from build123d import *

# Parameters (mm, degrees)
MODEL_R         = 9.4
MODEL_R_2       = 2.5
EXTRUDE_1_DEPTH = 6
SKETCH_2_W      = 6.222861065
SKETCH_2_H      = 6.222861065
SKETCH_2_W_2    = 12
SKETCH_2_H_2    = 6
SKETCH_2_W_3    = 11.79
SKETCH_2_H_3    = 6.29
SKETCH_2_W_4    = 6.039723033
SKETCH_2_H_4    = 6.178960273
SKETCH_2_H_5    = 12
SKETCH_2_W_5    = 6
SKETCH_2_H_6    = 6.764977387
EXTRUDE_2_DEPTH = 2


with BuildPart() as part:
    # Model → 凸台-拉伸1 (new body)
    with BuildSketch(Plane.XY):
        Polygon((1072.862228674, 1168.347447046), (1072.862228674, 1127.547447046), (1012.463824187, 1127.108430595), (1012.463824187, 1167.908430595), align=None)
        with Locations((1022.862228674, 1157.847447046)):
            Circle(MODEL_R, mode=Mode.SUBTRACT)
        with Locations((1042.662228674, 1157.847447046)):
            Circle(MODEL_R, mode=Mode.SUBTRACT)
        with Locations((1062.462228674, 1157.847447046)):
            Circle(MODEL_R, mode=Mode.SUBTRACT)
        with Locations((1022.862228674, 1138.047447046)):
            Circle(MODEL_R, mode=Mode.SUBTRACT)
        with Locations((1042.662228674, 1138.047447046)):
            Circle(MODEL_R, mode=Mode.SUBTRACT)
        with Locations((1062.462228674, 1138.047447046)):
            Circle(MODEL_R, mode=Mode.SUBTRACT)
        with Locations((1032.762228674, 1147.947447046)):
            Circle(MODEL_R_2, mode=Mode.SUBTRACT)
        with Locations((1052.562228674, 1147.947447046)):
            Circle(MODEL_R_2, mode=Mode.SUBTRACT)
    extrude(amount=EXTRUDE_1_DEPTH)

    # 草图2 → 凸台-拉伸2 (add)
    with BuildSketch(Plane.XY.offset(6)):
        with Locations((1015.57525472, 1164.797000063)):
            Rectangle(SKETCH_2_W, SKETCH_2_H)
        Polygon((1072.862228674, 1133.328066092), (1072.862228674, 1127.547447046), (1066.822505641, 1127.503546254), (1066.822505641, 1133.328066092), align=None)
        with Locations((1032.763038583, 1164.944548481)):
            Rectangle(SKETCH_2_W_2, SKETCH_2_H_2)
        with Locations((1052.562228674, 1165.088462385)):
            Rectangle(SKETCH_2_W_3, SKETCH_2_H_3)
        with Locations((1069.842367158, 1165.214066118)):
            Rectangle(SKETCH_2_W_4, SKETCH_2_H_4)
        with Locations((1032.762228674, 1147.947447046)):
            Rectangle(SKETCH_2_W_2, SKETCH_2_H_5)
        with Locations((1052.562228674, 1147.947447046)):
            Rectangle(SKETCH_2_W_2, SKETCH_2_H_5)
        with Locations((1069.842367158, 1147.947447046)):
            Rectangle(SKETCH_2_W_4, SKETCH_2_H_5)
        with Locations((1015.796351171, 1147.726326037)):
            Rectangle(SKETCH_2_W_5, SKETCH_2_H_5)
        Polygon((1058.457228674, 1127.45), (1058.457228674, 1133.509189688), (1046.667228674, 1133.509189688), (1046.667228674, 1127.38), align=None)
        Polygon((1038.763038583, 1127.3), (1038.763038583, 1133.508103592), (1026.763038583, 1133.508103592), (1026.763038583, 1127.22), align=None)
        with Locations((1015.57525472, 1130.493598172)):
            Rectangle(SKETCH_2_W, SKETCH_2_H_6)
    extrude(amount=EXTRUDE_2_DEPTH)


solid = part.part
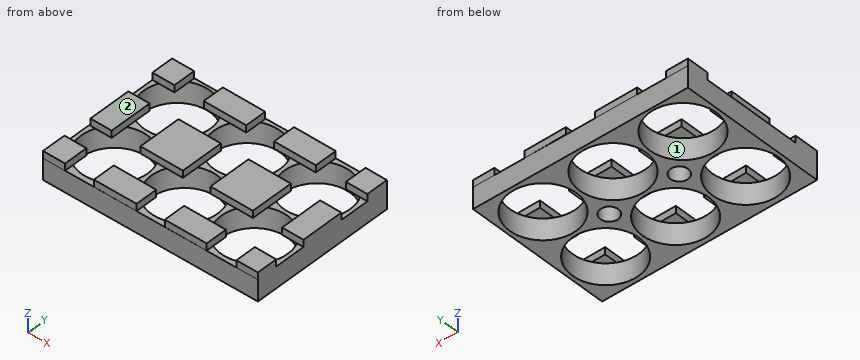
CAD build for the part. Positions are in the model's coordinates, mm. Face numbers are marked on the shaded views. A direction names the side the tool comes from. Round coordinates to 2 decimals unless told otherwise and drop trailing zeros. Write each loop counter-clockwise with the first axis right and the second up, starting at its lowest first coordinate (ties: lowest second). Pieces come first, ordered by that corner, then holes.
(1) Drop flat-ended pins along their axis: P1, Ø1, axis at x = 1033.5, y = 1137.5, coming from the +Z side; P2, Ø1.6, axis at x = 1054, z = 7, coming from the +Y side; P3, Ø3, axis at x = 1043.5, z = 6, coming from the +Y side. Give the stop position or say it passes through.
(2) 3-axis set-ups, long thin cutter, end or side, ignore diameter. For the marked faces 1 and 2: which of +Z, -Z, +X, -X, +Y, -Y reach the whole face in a straight line?
(3) Slice it at A-A, the plane y = 1155.5. Write the cut outline in (x, z).
(4) Slice it at C-C, the plane z = 4.5. Count the separate pieces of the cut face and the enclosed holes in it, and give its area (3 significant figures).
(5) Probe line 1 along X through (y, z) = (1162.5, 6.5); line 2 along X through (y, z) = (1154, 0.75); line 3 along Y through (x, z) = (1054.5, 6.25). List the from-to ranges inside material, lowest first.
(6) Slice it at D-D, the plane y = 1164.5. Write the cut outline in (x, z), and give its area (3 significant figures).
(7) Slice it at B-B, the plane x = 1045. Write the cut outline in (y, z).
From the geometry:
1. P1: stops at z = 6
1. P2: stops at y = 1168.23
1. P3: stops at y = 1168.14
2. face 1: -Z
2. face 2: +Z, +X, -X, +Y, -Y
3. outline: (1012.46, 0) - (1013.76, 0) - (1013.76, 6) - (1012.46, 6) - close; (1031.96, 0) - (1033.56, 0) - (1033.56, 6) - (1031.96, 6) - close; (1051.76, 0) - (1053.36, 0) - (1053.36, 6) - (1051.76, 6) - close; (1071.56, 0) - (1072.86, 0) - (1072.86, 6) - (1071.56, 6) - close
4. separate pieces: 1
4. enclosed holes: 8
4. area: 759 mm2
5. line 1: x = 1012.46 to 1018.69, 1026.76 to 1038.76, 1046.67 to 1058.46, 1066.82 to 1072.86
5. line 2: x = 1012.46 to 1014.29, 1031.44 to 1034.09, 1051.24 to 1053.89, 1071.04 to 1072.86
5. line 3: y = 1127.43 to 1133.51, 1141.95 to 1153.95, 1161.94 to 1168.23
6. outline: (1012.46, 0) - (1016.22, 0) - (1016.22, 6) - (1018.69, 6) - (1018.69, 8) - (1012.46, 8) - close; (1026.76, 6) - (1029.5, 6) - (1029.5, 0) - (1036.02, 0) - (1036.02, 6) - (1038.76, 6) - (1038.76, 8) - (1026.76, 8) - close; (1046.67, 6) - (1049.3, 6) - (1049.3, 0) - (1055.82, 0) - (1055.82, 6) - (1058.46, 6) - (1058.46, 8) - (1046.67, 8) - close; (1066.82, 6) - (1069.1, 6) - (1069.1, 0) - (1072.86, 0) - (1072.86, 8) - (1066.82, 8) - close
6. area: 195 mm2
7. outline: (1127.34, 0) - (1128.94, 0) - (1128.94, 6) - (1127.34, 6) - close; (1147.15, 0) - (1148.74, 0) - (1148.74, 6) - (1147.15, 6) - close; (1166.95, 0) - (1168.14, 0) - (1168.14, 6) - (1166.95, 6) - close
